Check sheet for the modelled part. Datum: model origin and axes. Units: mm. A direction names the side the tool comes from. Round coordinates to 2 decimals unless told otherwise and drop trailing zeros. Write each loop counter-clockwise with the first axis right and the second up, starting at its lowest first coordinate (ties: lowest second). Pieces come first, ordered by that corner, then holes.
from build123d import *

# Parameters (mm, degrees)
SKETCH1_R                       = 3.6
SKETCH1_R_2                     = 2.5
BOSS_EXTRUDE1_DEPTH             = 1.25
FILLET1_R                       = 5
FILLET2_R                       = 10
CUT_EXTRUDE1_DEPTH              = 60.720704115
FILLET3_R                       = 0.5
SKETCH3_R                       = 2.65
BOSS_EXTRUDE2_DEPTH             = 4.5
M3X0_5_TAPPED_HOLE1_D           = 2.5
M3X0_5_TAPPED_HOLE1_DEPTH       = 6
M3X0_5_TAPPED_HOLE1_CSINK_D     = 3.5
M3X0_5_TAPPED_HOLE1_CSINK_ANGLE = 90
M3X0_5_TAPPED_HOLE1_TIP         = 0.751075774
SKETCH7_R                       = 2.625
BOSS_EXTRUDE3_DEPTH             = 1.5
M3X0_5_TAPPED_HOLE2_D           = 2.5
M3X0_5_TAPPED_HOLE2_CSINK_D     = 3.5
M3X0_5_TAPPED_HOLE2_CSINK_ANGLE = 90


with BuildPart() as part:
    # Sketch1 → Boss-Extrude1 (new, symmetric)
    with BuildSketch(Plane.XY):
        with BuildLine():
            Line((-0.5, -27.75), (-0.5, -23.75))
            Line((-0.5, -23.75), (44.5, -23.75))
            Line((44.5, -23.75), (44.5, 23.75))
            Line((44.5, 23.75), (-44.5, 23.75))
            Line((-44.5, 23.75), (-44.5, -23.75))
            Line((-44.5, -23.75), (-24.5, -23.75))
            Line((-24.5, -23.75), (-24.5, -27.75))
            ThreePointArc((-24.5, -27.75), (-12.5, -39.75), (-0.5, -27.75))
        make_face()
        with Locations((-12.5, -27.85)):
            Circle(SKETCH1_R, mode=Mode.SUBTRACT)
        with Locations((7.5, 11.75)):
            Circle(SKETCH1_R_2, mode=Mode.SUBTRACT)
        with Locations((-32.5, 11.75)):
            Circle(SKETCH1_R_2, mode=Mode.SUBTRACT)
    extrude(amount=BOSS_EXTRUDE1_DEPTH, both=True)

    # Fillet1
    fillet1_edges = [part.edges().sort_by_distance(p)[0] for p in [
        (44.5, -23.75, 0),
        (-44.5, -23.75, 0),
    ]]
    fillet(fillet1_edges, radius=FILLET1_R)

    # Fillet2
    fillet2_edges = [part.edges().sort_by_distance(p)[0] for p in [
        (-44.5, 23.75, 0),
        (44.5, 23.75, 0),
    ]]
    fillet(fillet2_edges, radius=FILLET2_R)

    # Sketch2 → Cut-Extrude1 (cut, through all)
    with BuildSketch(Plane.XY.offset(1.25)):
        with BuildLine():
            Line((18.5, -23.75), (21.5, -23.75))
            Line((21.5, -23.75), (21.5, 4.75))
            ThreePointArc((21.5, 4.75), (20, 6.25), (18.5, 4.75))
            Line((18.5, 4.75), (18.5, -23.75))
        make_face()
        Polygon((44.5, -0.75), (38, -0.75), (38, -12.75), (39.75, -12.75), (39.75, -2.5), (44.5, -2.5), align=None)
        Polygon((-38, -12.75), (-39.75, -12.75), (-39.75, -2.5), (-44.5, -2.5), (-44.5, -0.75), (-38, -0.75), align=None)
    extrude(amount=-CUT_EXTRUDE1_DEPTH, mode=Mode.SUBTRACT)

    # Fillet3
    fillet3_edges = [part.edges().sort_by_distance(p)[0] for p in [
        (-0.5, -23.75, 0),
        (-24.5, -23.75, 0),
        (44.5, -0.75, 0),
        (44.5, -2.5, 0),
        (39.75, -2.5, 0),
        (39.75, -12.75, 0),
        (38, -12.75, 0),
        (38, -0.75, 0),
        (-38, -0.75, 0),
        (-38, -12.75, 0),
        (-39.75, -12.75, 0),
        (-39.75, -2.5, 0),
        (-44.5, -2.5, 0),
        (-44.5, -0.75, 0),
        (18.5, -23.75, 0),
        (21.5, -23.75, 0),
    ]]
    fillet(fillet3_edges, radius=FILLET3_R)

    # Sketch3 → Boss-Extrude2 (add)
    with BuildSketch(Plane.XY.offset(1.25)):
        with Locations((11, -0.75)):
            Circle(SKETCH3_R)
        with Locations((-3, -0.75)):
            Circle(SKETCH3_R)
    extrude(amount=BOSS_EXTRUDE2_DEPTH)

    # M3x0.5 Tapped Hole1
    with Locations(Plane.XY.offset(5.75)):
        with Locations((-3, -0.75), (11, -0.75)):
            CounterSinkHole(M3X0_5_TAPPED_HOLE1_D / 2, M3X0_5_TAPPED_HOLE1_CSINK_D / 2, depth=M3X0_5_TAPPED_HOLE1_DEPTH, counter_sink_angle=M3X0_5_TAPPED_HOLE1_CSINK_ANGLE)
            with Locations((0, 0, -(M3X0_5_TAPPED_HOLE1_DEPTH + M3X0_5_TAPPED_HOLE1_TIP / 2))):  # 118° drill point
                Cone(0, M3X0_5_TAPPED_HOLE1_D / 2, M3X0_5_TAPPED_HOLE1_TIP, mode=Mode.SUBTRACT)

    # Sketch7 → Boss-Extrude3 (add)
    with BuildSketch(Plane(origin=(0, 0, -1.25), x_dir=(-1, 0, 0), z_dir=(0, 0, -1))):
        with Locations(Location((13.375, 9.5, 0), (0, 0, 180))):
            Circle(SKETCH7_R)
        with Locations(Location((31.375, -8.5, 0), (0, 0, 180))):
            Circle(SKETCH7_R)
    extrude(amount=BOSS_EXTRUDE3_DEPTH)

    # M3x0.5 Tapped Hole2 (through all)
    with Locations(Plane(origin=(0, 0, -2.75), x_dir=(-1, 0, 0), z_dir=(0, 0, -1))):
        with Locations((13.375, 9.5), (31.375, -8.5)):
            CounterSinkHole(M3X0_5_TAPPED_HOLE2_D / 2, M3X0_5_TAPPED_HOLE2_CSINK_D / 2, counter_sink_angle=M3X0_5_TAPPED_HOLE2_CSINK_ANGLE)


solid = part.part
1. Scan lines: line 1 along X through (y, z) = (-8.5, -0.2) (3 decimals); line 2 along X through (y, z) = (9.5, -0.3) (3 decimals); line 3 along Y through (x, z) = (6, -0.5). Record each from-to range of solid material in increasing order.
2. Sectioned sample at D-D, the plane x = 3.5. Enter the section's corners in (y, z), plus the area to 3 significant figures.
3. Sectioned sample at C-C, the plane y = -8.5. Enter the section's corners in (x, z) (3 decimals).
4. Sectioned sample at A-A, the plane y = -17. Enter the section's corners in (x, z), plus the area to 3 significant figures.
5. Release check for a two-part mould opening along X. For faces 6 (the conical face through (11.2, -0.83, -0.87)), 7 (the flat face through (41, -0.75, 0)), 8 (the flat face through (44.5, 7, 0)) record: released by +X, released by -X, zero draft, split by the parting line, or undercut.
6. Set-up check for faces 1 (the flat face through (21.5, -9, 0)), 2 (the cylindrical face through (-34, -8.6, -2)), 3 (the cylindrical face through (-3.57, -3.34, 3.47)), 4 (the flat face through (-24.5, -26, 0)), 5 (the flat face through (38, -7, 0)): record each of +Z, -Z, +X, -X, +Y, -Y from which the full face is reachable in a straight line by a thin tool's end or side.
7. Sectioned sample at B-B, the plane z = 2.5. Enter the section's corners in (x, y), plus the area to 3 significant figures.
8. Go/stop test with flat-tipped pins: pin 1 (1.5 mm diameter, centred on x = 9, z = 1, fed in from -Y); pin 2 (6 mm diameter, centred on x = -24.5, y = -20, fed in from +Z); pin 3 (19 mm diameter, centred on x = 21, y = -11.5, fed in from -Z). Record where each tip stops, or that it passes through.
Computed values:
1. line 1: x = -44.5 to -39.75, -38 to -32.625, -30.125 to 18.5, 21.5 to 38, 39.75 to 44.5
1. line 2: x = -44.5 to -33.59, -31.41 to -14.625, -12.125 to 6.41, 8.59 to 44.5
1. line 3: y = -23.75 to 9.75, 13.75 to 23.75
2. outline: (-23.75, -1.25) - (23.75, -1.25) - (23.75, 1.25) - (-23.75, 1.25) - close
2. area: 119 mm2
3. outline: (-44.5, -1.25) - (-39.75, -1.25) - (-39.75, 1.25) - (-44.5, 1.25) - close; (-38, -1.25) - (-34, -1.25) - (-34, -2.75) - (-33.125, -2.75) - (-32.625, -2.25) - (-32.625, 1.25) - (-38, 1.25) - close; (-30.125, -2.25) - (-29.625, -2.75) - (-28.75, -2.75) - (-28.75, -1.25) - (18.5, -1.25) - (18.5, 1.25) - (-30.125, 1.25) - close; (21.5, -1.25) - (38, -1.25) - (38, 1.25) - (21.5, 1.25) - close; (39.75, -1.25) - (44.5, -1.25) - (44.5, 1.25) - (39.75, 1.25) - close
4. outline: (-44.5, -1.25) - (18.5, -1.25) - (18.5, 1.25) - (-44.5, 1.25) - close; (21.5, -1.25) - (44.5, -1.25) - (44.5, 1.25) - (21.5, 1.25) - close
4. area: 215 mm2
5. face 6: undercut
5. face 7: zero draft
5. face 8: released by +X
6. face 1: +Z, -Z, -Y
6. face 2: -Z
6. face 3: +Z
6. face 4: +Z, -Z, -X, -Y
6. face 5: +Z, -Z
7. outline: circle Ø5.3 at (-3, -0.75); circle Ø5.3 at (11, -0.75); hole circle Ø2.5 at (-3, -0.75); hole circle Ø2.5 at (11, -0.75)
7. area: 34.3 mm2
8. pin 1: stops at y = -23.75
8. pin 2: stops at z = 1.25
8. pin 3: stops at z = -1.25
